Part model, mm, in its own coordinate system. Face numbers are marked on the shaded views. Coordinates: 2 decimals unless noted, no trailing zeros. Order: outer loops, then holes, each group sorted by start corner. A loop starts at its lowest first (then second) coordinate and runs counter-clockwise, first axis right, second up. Notation, with made-up numbers: M 79.5,34.25 L 121.5,34.25 A23 ccw 121.5,42.25 Z; hole C 32.25,85 d7. An arc over 180 degrees is marked long. Write item = value, one per line. Start each with the question number.
from build123d import *

# Parameters (mm, degrees)
SKETCH_1_W          = 140
SKETCH_1_H          = 75
EXTRUDE_1_DEPTH     = 2
SKETCH_2_W          = 4
SKETCH_2_H          = 52
EXTRUDE_2_DEPTH     = 18
SKETCH_3_R          = 1.55
CUT_EXTRUDE_1_DEPTH = 15
SKETCH_5_R          = 1.55
CUT_EXTRUDE_2_DEPTH = 15


with BuildPart() as part:
    # 草图1 → 凸台-拉伸1 (new body)
    with BuildSketch(Plane(origin=(0, 0, 0), x_dir=(1, 0, 0), z_dir=(0, 1, 0))):
        Rectangle(SKETCH_1_W, SKETCH_1_H)
    extrude(amount=EXTRUDE_1_DEPTH)

    # 草图2 → 凸台-拉伸2 (add)
    with BuildSketch(Plane(origin=(0, 2, 0), x_dir=(1, 0, 0), z_dir=(0, 1, 0))):
        with Locations((58.5, 0)):
            Rectangle(SKETCH_2_W, SKETCH_2_H)
        with Locations((-58.5, 0)):
            Rectangle(SKETCH_2_W, SKETCH_2_H)
    extrude(amount=EXTRUDE_2_DEPTH)

    # 草图3 → 切除-拉伸1 (cut)
    with BuildSketch(Plane.ZY.offset(60.5)):
        with Locations((-14.5, 12.5)):
            Circle(SKETCH_3_R)
        with Locations((14.5, 12.5)):
            Circle(SKETCH_3_R)
    cut_extrude_1 = extrude(amount=-CUT_EXTRUDE_1_DEPTH, mode=Mode.SUBTRACT)

    # 镜向1: 切除-拉伸1 across plane
    add(cut_extrude_1.mirror(Plane(origin=(0, 0, 0), x_dir=(0, 0, 1), z_dir=(1, 0, 0))), mode=Mode.SUBTRACT)

    # 草图5 → 切除-拉伸2 (cut)
    with BuildSketch(Plane(origin=(0, 0, 0), x_dir=(-1, 0, 0), z_dir=(0, -1, 0))):
        with Locations(Location((0, -10.5, 0), (0, 0, 90))):
            Circle(SKETCH_5_R)
        with Locations(Location((-10.5, 0, 0), (0, 0, 90))):
            Circle(SKETCH_5_R)
        with Locations(Location((10.5, 0, 0), (0, 0, 90))):
            Circle(SKETCH_5_R)
        with Locations(Location((0, 10.5, 0), (0, 0, 90))):
            Circle(SKETCH_5_R)
    extrude(amount=-CUT_EXTRUDE_2_DEPTH, mode=Mode.SUBTRACT)


solid = part.part
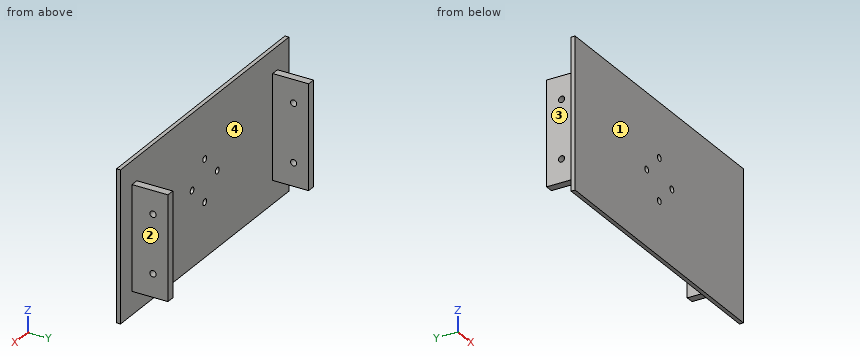
Item 1: Cut at C-C, the plane z = 10.5. Write the cut outline in (x, y), and give its area (3 significant figures).
Item 2: Pull direction X, two halves, no side cores. Call the marked faces 1, 2, 3 and 4: pulls with the +X half, pulls with the -X half, needs draft (parallel to the pull), parting line crosses it, or undercut.
Item 3: Cut at D-D, the plane y = 8.75. Write the cut outline in (x, z), and give its area (3 significant figures).
Item 4: Cut at B-B, the plane x = -59. Write the cut outline in (y, z), and give its area (3 significant figures).
Item 5: Flat gauge pins, fed straight in: pin 1 (2 mm diameter, centred on x = 59, y = 11.5, fed in from +Z); pin 2 (1.5 mm diameter, centred on y = 8.5, z = -16, fed in from -X); pin 3 (6 mm diameter, centred on x = 51, z = -20.5, fed in from +Y). Where does each tip first touch, or does it go through?
Item 6: Wall check: line 1 along X through (y, z) = (1.5, 0); line 2 along X through (y, z) = (13.25, 19); line 3 along Z through (x, y) = (59.4, 12.5). Give the ranges that are in metal, low to high. Write a range as [from, to].
Item 7: Cut at A-A, the plane z = -14.5. Write the cut outline in (x, y), and give its area (3 significant figures).
Filled sheet:
q1.outline = M -70,0 L -1.55,0 L -1.55,2 L -56.5,2 L -56.5,20 L -60.5,20 L -60.5,2 L -70,2 Z; M 1.55,0 L 70,0 L 70,2 L 60.5,2 L 60.5,20 L 56.5,20 L 56.5,2 L 1.55,2 Z
q1.area = 418 mm2
q2.face_1 = needs draft
q2.face_2 = pulls with the +X half
q2.face_3 = pulls with the -X half
q2.face_4 = undercut
q3.outline = M -60.5,-26 L -56.5,-26 L -56.5,26 L -60.5,26 Z; M 56.5,-26 L 60.5,-26 L 60.5,26 L 56.5,26 Z
q3.area = 416 mm2
q4.outline = M 0,-37.5 L 2,-37.5 L 2,-26 L 20,-26 L 20,26 L 2,26 L 2,37.5 L 0,37.5 Z; hole C 12.5,-14.5 d3.1; hole C 12.5,14.5 d3.1
q4.area = 1,070 mm2
q5.pin_1 = 26
q5.pin_2 = -60.5
q5.pin_3 = 2
q6.line_1 = [-70, -12.05], [-8.95, 8.95], [12.05, 70]
q6.line_2 = [-60.5, -56.5], [56.5, 60.5]
q6.line_3 = [-26, -16.05], [-12.95, 12.95], [16.05, 26]
q7.outline = M -70,0 L 70,0 L 70,2 L 60.5,2 L 60.5,10.95 L 56.5,10.95 L 56.5,2 L -56.5,2 L -56.5,10.95 L -60.5,10.95 L -60.5,2 L -70,2 Z; M -60.5,14.05 L -56.5,14.05 L -56.5,20 L -60.5,20 Z; M 56.5,14.05 L 60.5,14.05 L 60.5,20 L 56.5,20 Z
q7.area = 399 mm2
